Part model, mm, in its own coordinate system. A direction names the side the tool comes from. Round coordinates to 2 decimals unless told otherwise and drop trailing zeros. Write each loop counter-clockwise with the first axis right and the second up, starting at its lowest first coordinate (ties: lowest second). Pieces come first, ordered by that corner, then holes.
1) Saw through at B-B on x = 36. Write the cut outline in (y, z).
2) Pull direction X, two halves, no side cores. Call faces 1 (the cylindrical face through (-8.486, -9.848, 0.597)), 2 (the flat face through (-19.5, -5.7, 0.4)), 3 (the cylindrical face through (-8.475, -11.143, 0.597)), 4 (the cylindrical face through (-4.336, -19.524, 0.597)): +X half, -X half, draft (parallel to the pull), parting line (faces both ways), or undercut.
3) Drill centre lines: L1, parallel to X at y = -12, z = 0.6; L2, parallel to Z at x = 27, y = -16.5; L3, parallel to Y at x = -5, z = 0.7. Where is each one in solid material? Low to high.
4) Which spindle directions (+Z, -Z, +X, -X, +Y, -Y) get a long thin tool onto all of the face, cutting with end or side? Do faces 5 (the flat face through (3, 11, 0.4)), 6 (the flat face through (-1, 0, 0)). Say none if no direction does.
5) Saw through at A-A on y = 16.5. Write the cut outline in (x, z), and give its area (3 significant figures).
6) Flat gauge pin, fed straight in: pin 1 (5 mm diameter, centred on x = 15.5, y = 20, fed in from +Z). Where does the tip first touch, or does it go through?
7) Saw through at C-C on x = -9.5. Write the cut outline in (y, z), and give its area (3 significant figures).
```python
from build123d import *

# Parameters (mm, degrees)
F0_W     = 85
F0_H     = 55
F1_DEPTH = 0.4
F2_R     = 20
F3_DEPTH = 0.4


with BuildPart() as f1:
    # F0 (on Top) → F1 (new body)
    with BuildSketch(Plane.XY):
        Rectangle(F0_W, F0_H)
    extrude(amount=F1_DEPTH)

    # F2 (on face) → F3 (join)
    with BuildSketch(Plane.XY.offset(0.4)):
        Circle(F2_R)
        with BuildLine():
            add(Edge.make_bspline(
                [(-7.4961080118, -5.409697216), (-8.0117330118, -4.399931591), (-8.0117330118, -3.032744091)],
                knots=[0, 0, 0, 1, 1, 1], degree=2))
            add(Edge.make_bspline(
                [(-8.0117330118, -3.032744091), (-8.0117330118, -0.938994091), (-6.8886861368, 0.2084668465)],
                knots=[0, 0, 0, 1, 1, 1], degree=2))
            add(Edge.make_bspline(
                [(-6.8886861368, 0.2084668465), (-5.7656392618, 1.355927784), (-3.7324361368, 1.355927784)],
                knots=[0, 0, 0, 1, 1, 1], degree=2))
            add(Edge.make_bspline(
                [(-3.7324361368, 1.355927784), (-2.3047017618, 1.355927784), (-1.4140767618, 0.873505909)],
                knots=[0, 0, 0, 1, 1, 1], degree=2))
            add(Edge.make_bspline(
                [(-1.4140767618, 0.873505909), (-0.5234517618, 0.391084034), (-0.0410298868, -0.671415966)],
                knots=[0, 0, 0, 1, 1, 1], degree=2))
            Line((-0.0410298868, -0.671415966), (-1.1523580118, -0.999540966))
            add(Edge.make_bspline(
                [(-1.1523580118, -0.999540966), (-1.5175923868, -0.267119091), (-2.1611470743, 0.0678418465)],
                knots=[0, 0, 0, 1, 1, 1], degree=2))
            add(Edge.make_bspline(
                [(-2.1611470743, 0.0678418465), (-2.8047017618, 0.402802784), (-3.7636861368, 0.402802784)],
                knots=[0, 0, 0, 1, 1, 1], degree=2))
            add(Edge.make_bspline(
                [(-3.7636861368, 0.402802784), (-5.2539205118, 0.402802784), (-6.0410298868, -0.497587841)],
                knots=[0, 0, 0, 1, 1, 1], degree=2))
            add(Edge.make_bspline(
                [(-6.0410298868, -0.497587841), (-6.8281392618, -1.397978466), (-6.8281392618, -3.032744091)],
                knots=[0, 0, 0, 1, 1, 1], degree=2))
            add(Edge.make_bspline(
                [(-6.8281392618, -3.032744091), (-6.8281392618, -4.661650341), (-5.9922017618, -5.605009716)],
                knots=[0, 0, 0, 1, 1, 1], degree=2))
            add(Edge.make_bspline(
                [(-5.9922017618, -5.605009716), (-5.1562642618, -6.548369091), (-3.6777486368, -6.548369091)],
                knots=[0, 0, 0, 1, 1, 1], degree=2))
            add(Edge.make_bspline(
                [(-3.6777486368, -6.548369091), (-2.8359517618, -6.548369091), (-2.1064595743, -6.292509716)],
                knots=[0, 0, 0, 1, 1, 1], degree=2))
            add(Edge.make_bspline(
                [(-2.1064595743, -6.292509716), (-1.3769673868, -6.036650341), (-0.9257955118, -5.597197216)],
                knots=[0, 0, 0, 1, 1, 1], degree=2))
            Line((-0.9257955118, -5.597197216), (-0.9257955118, -4.046415966))
            Line((-0.9257955118, -4.046415966), (-3.4961080118, -4.046415966))
            Line((-3.4961080118, -4.046415966), (-3.4961080118, -3.069853466))
            Line((-3.4961080118, -3.069853466), (0.1484232382, -3.069853466))
            Line((0.1484232382, -3.069853466), (0.1484232382, -6.036650341))
            add(Edge.make_bspline(
                [(0.1484232382, -6.036650341), (-0.5351705118, -6.731962841), (-1.5273580118, -7.1137987785)],
                knots=[0, 0, 0, 1, 1, 1], degree=2))
            add(Edge.make_bspline(
                [(-1.5273580118, -7.1137987785), (-2.5195455118, -7.495634716), (-3.6777486368, -7.495634716)],
                knots=[0, 0, 0, 1, 1, 1], degree=2))
            add(Edge.make_bspline(
                [(-3.6777486368, -7.495634716), (-5.0273580118, -7.495634716), (-6.0039205118, -6.9575487785)],
                knots=[0, 0, 0, 1, 1, 1], degree=2))
            add(Edge.make_bspline(
                [(-6.0039205118, -6.9575487785), (-6.9804830118, -6.419462841), (-7.4961080118, -5.409697216)],
                knots=[0, 0, 0, 1, 1, 1], degree=2))
        make_face(mode=Mode.SUBTRACT)
        with BuildLine():
            ThreePointArc((13.716509354, 2.803100273), (-8.8531518731, -10.845353932), (0, 14))
            Line((0, 14), (0, 13))
            ThreePointArc((0, 13), (-8.1412436535, -10.135095055), (12.6941966607, 2.803100273))
            Line((12.6941966607, 2.803100273), (13.716509354, 2.803100273))
        make_face(mode=Mode.SUBTRACT)
        with BuildLine():
            add(Edge.make_bspline(
                [(7.744643158, 13.2869364135), (7.082533783, 13.6834207885), (6.172377533, 13.6834207885)],
                knots=[0, 0, 0, 1, 1, 1], degree=2))
            add(Edge.make_bspline(
                [(6.172377533, 13.6834207885), (4.744643158, 13.6834207885), (3.9506978455, 12.7654520385)],
                knots=[0, 0, 0, 1, 1, 1], degree=2))
            add(Edge.make_bspline(
                [(3.9506978455, 12.7654520385), (3.156752533, 11.8474832885), (3.156752533, 10.2478739135)],
                knots=[0, 0, 0, 1, 1, 1], degree=2))
            add(Edge.make_bspline(
                [(3.156752533, 10.2478739135), (3.156752533, 8.6677957885), (3.9839009705, 7.705881726)],
                knots=[0, 0, 0, 1, 1, 1], degree=2))
            add(Edge.make_bspline(
                [(3.9839009705, 7.705881726), (4.811049408, 6.7439676635), (6.221205658, 6.7439676635)],
                knots=[0, 0, 0, 1, 1, 1], degree=2))
            add(Edge.make_bspline(
                [(6.221205658, 6.7439676635), (8.027846283, 6.7439676635), (8.938002533, 8.5330301635)],
                knots=[0, 0, 0, 1, 1, 1], degree=2))
            Line((8.938002533, 8.5330301635), (9.889174408, 8.0564676635))
            add(Edge.make_bspline(
                [(9.889174408, 8.0564676635), (9.357924408, 6.9451395385), (8.396986908, 6.3650614135)],
                knots=[0, 0, 0, 1, 1, 1], degree=2))
            add(Edge.make_bspline(
                [(8.396986908, 6.3650614135), (7.436049408, 5.7849832885), (6.166518158, 5.7849832885)],
                knots=[0, 0, 0, 1, 1, 1], degree=2))
            add(Edge.make_bspline(
                [(6.166518158, 5.7849832885), (4.865736908, 5.7849832885), (3.916518158, 6.3259989135)],
                knots=[0, 0, 0, 1, 1, 1], degree=2))
            add(Edge.make_bspline(
                [(3.916518158, 6.3259989135), (2.967299408, 6.8670145385), (2.4702290955, 7.8709207885)],
                knots=[0, 0, 0, 1, 1, 1], degree=2))
            add(Edge.make_bspline(
                [(2.4702290955, 7.8709207885), (1.973158783, 8.8748270385), (1.973158783, 10.2478739135)],
                knots=[0, 0, 0, 1, 1, 1], degree=2))
            add(Edge.make_bspline(
                [(1.973158783, 10.2478739135), (1.973158783, 12.3045145385), (3.084486908, 13.4705301635)],
                knots=[0, 0, 0, 1, 1, 1], degree=2))
            add(Edge.make_bspline(
                [(3.084486908, 13.4705301635), (4.195815033, 14.6365457885), (6.160658783, 14.6365457885)],
                knots=[0, 0, 0, 1, 1, 1], degree=2))
            add(Edge.make_bspline(
                [(6.160658783, 14.6365457885), (7.533705658, 14.6365457885), (8.455580658, 14.0994364135)],
                knots=[0, 0, 0, 1, 1, 1], degree=2))
            add(Edge.make_bspline(
                [(8.455580658, 14.0994364135), (9.377455658, 13.5623270385), (9.811049408, 12.5056864135)],
                knots=[0, 0, 0, 1, 1, 1], degree=2))
            Line((9.811049408, 12.5056864135), (8.705580658, 12.1404520385))
            add(Edge.make_bspline(
                [(8.705580658, 12.1404520385), (8.406752533, 12.8904520385), (7.744643158, 13.2869364135)],
                knots=[0, 0, 0, 1, 1, 1], degree=2))
        make_face(mode=Mode.SUBTRACT)
    extrude(amount=F3_DEPTH)


solid = f1.part
```
Completed:
1. outline: (-27.5, 0) - (27.5, 0) - (27.5, 0.4) - (-27.5, 0.4) - close
2. face 1: undercut
2. face 2: draft
2. face 3: undercut
2. face 4: parting line
3. L1: x = -16 to -7.21, -5 to 5, 7.21 to 16
3. L2: z = 0 to 0.4
3. L3: y = -19.36 to -13.08, -12 to -7.35, -6.31 to 0.21, 1.23 to 12, 13.08 to 19.36
4. face 5: +Z
4. face 6: -Z, +X, -X, +Y, -Y
5. outline: (-42.5, 0) - (42.5, 0) - (42.5, 0.4) - (11.3, 0.4) - (11.3, 0.8) - (-11.3, 0.8) - (-11.3, 0.4) - (-42.5, 0.4) - close
5. area: 43.0 mm2
6. pin 1: stops at z = 0.4
7. outline: (-27.5, 0) - (27.5, 0) - (27.5, 0.4) - (17.6, 0.4) - (17.6, 0.8) - (10.28, 0.8) - (10.28, 0.4) - (8.87, 0.4) - (8.87, 0.8) - (-8.87, 0.8) - (-8.87, 0.4) - (-10.28, 0.4) - (-10.28, 0.8) - (-17.6, 0.8) - (-17.6, 0.4) - (-27.5, 0.4) - close
7. area: 35.0 mm2
